from build123d import *

# Parameters (mm, degrees)
SKETCH1_W               = 552.45
SKETCH1_H               = 19.05
BOSS_EXTRUDE1_DEPTH     = 6.35
CUT_EXTRUDE1_DEPTH      = 277.680802099
CUT_EXTRUDE1_DEPTH_BACK = 277.680802099
SKETCH2_R               = 5.588
FILLET1_R               = 2.54


with BuildPart() as part:
    # Sketch1 → Boss-Extrude1 (new, symmetric)
    with BuildSketch(Plane.XY):
        Rectangle(SKETCH1_W, SKETCH1_H)
    extrude(amount=BOSS_EXTRUDE1_DEPTH, both=True)

    # Sketch2 → Cut-Extrude1 (cut, two sides: drawn at the far end of the back side and taken through both)
    with BuildSketch(Plane.XY.offset(6.35).offset(-CUT_EXTRUDE1_DEPTH_BACK)):
        Circle(SKETCH2_R)
        with Locations((250.825, 0)):
            Circle(SKETCH2_R)
        with Locations((-250.825, 0)):
            Circle(SKETCH2_R)
    extrude(amount=CUT_EXTRUDE1_DEPTH + CUT_EXTRUDE1_DEPTH_BACK, mode=Mode.SUBTRACT)

    # Fillet1
    fillet1_edges = [part.edges().sort_by_distance(p)[0] for p in [
        (-276.225, 0, 6.35),
        (276.225, 0, 6.35),
        (-276.225, 0, -6.35),
        (276.225, 0, -6.35),
    ]]
    fillet(fillet1_edges, radius=FILLET1_R)


solid = part.part
Can you work these out from the model? Positions are in its coordinate system, mm. Give positions to 0.01 mm unless a question says otherwise; leave off trailing zeros. Order: outer loops, then holes, each group sorted by start corner. A loop starts at its lowest first (then second) coordinate and runs counter-clockwise, first axis right, second up. Notation, with made-up numbers: M 14.5,68 L 39.5,68 A14 ccw 39.5,74 Z; hole C 2,2 d8. An arc over 180 degrees is marked long. Use a Markdown table: item, result. Add a question column.
Item 1: Suppose I cut it at A-A (x = 0). List the corners of the cut face in (y, z) for me (3 decimals).
Item 2: If I drill on L1, parallel to X at y = 0, z = -3.25 (3 decimals); L2, parallel to X at y = 2.75, z = 1.5 (3 decimals); L3, parallel to Y at x = 0, z = -0.5 (3 decimals), over which ranges is the centre line in solid material (lowest first)? Write a range as [from, to].
Item 3: Will this pin go through, and if not, where does the flat tip stop? pin 1 (6.5 mm diameter, centred on x = 250.825, y = 0, fed in from +Z).
Item 4: Suppose I cut it at C-C (z = 0.75). List the corners of the cut face in (x, y) for me (3 decimals), then the cut area to 3 significant figures.
Item 5: We'd pull the mould along X, two halves only. Please class faces 1 (the cylindrical face through (-4.434, -3.4, -0.089)), 2 (the flat face through (-3.8, 4.4, 6.35)): +X half, -X half, draft (parallel to the pull), parting line (faces both ways), or undercut.
Item 6: Suppose I cut it at B-B (y = 0). List the corners of the cut face in (x, z) for me (3 decimals), then the cut area to 3 significant figures.
Answer sheet:
| question | item | result |
|---|---|---|
| 1 | outline | M -9.525,-6.35 L -5.588,-6.35 L -5.588,6.35 L -9.525,6.35 Z; M 5.588,-6.35 L 9.525,-6.35 L 9.525,6.35 L 5.588,6.35 Z |
| 2 | L1 | x = [-276.225, -256.413], [-245.237, -5.588], [5.588, 245.237], [256.413, 276.225] |
| 2 | L2 | x = [-276.225, -255.689], [-245.961, -4.864], [4.864, 245.961], [255.689, 276.225] |
| 2 | L3 | y = [-9.525, -5.588], [5.588, 9.525] |
| 3 | pin 1 | passes through |
| 4 | outline | M -276.225,-9.525 L 276.225,-9.525 L 276.225,9.525 L -276.225,9.525 Z; hole C -250.825,0 d11.176; hole C 0,0 d11.176; hole C 250.825,0 d11.176 |
| 4 | area | 10,200 mm² |
| 5 | face 1 | undercut |
| 5 | face 2 | draft |
| 6 | outline | M -276.225,-3.81 A2.54 ccw -273.685,-6.35 L -256.413,-6.35 L -256.413,6.35 L -273.685,6.35 A2.54 ccw -276.225,3.81 Z; M -245.237,-6.35 L -5.588,-6.35 L -5.588,6.35 L -245.237,6.35 Z; M 5.588,-6.35 L 245.237,-6.35 L 245.237,6.35 L 5.588,6.35 Z; M 256.413,-6.35 L 273.685,-6.35 A2.54 ccw 276.225,-3.81 L 276.225,3.81 A2.54 ccw 273.685,6.35 L 256.413,6.35 Z |
| 6 | area | 6,580 mm² |
